Here's how the part is built. I have some questions about the finished solid (model axes, mm). Coordinates: 2 decimals unless noted, no trailing zeros. Write each loop counter-clockwise with the first axis right and the second up, starting at its lowest first coordinate (ties: lowest second). Pieces come first, ordered by that corner, then holes. Notation, with made-up numbers: M -24,56.25 L -13,56.25 A18 ccw -13,75.25 Z; hole C 31,32.5 d1. An arc over 180 degrees is marked long. Use one line per item in the form item = value. Start each with the question number.
1. I want a section at B-B, the plane y = 11. List the corners of the cut face in (x, z) for me.
2. I want a section at A-A, the plane x = 5. List the corners of the cut face in (y, z) for me, plus the area to 3 significant figures.
3. I want a section at C-C, the plane z = 2.5. List the corners of the cut face in (x, y) for me, plus the area to 3 significant figures.
4. I'm going to push a flat-ended pin straight in: pin 1 Ø3.5 at (y, z) = (5.5, 5) entering from +X. Where does the tip first touch, or does it pass through?
5. I want a section at D-D, the plane y = 7. List the corners of the cut face in (x, z) for me.
6. Please list where these lines run through material, in increasing order: line 1 along Y through (x, z) = (5, 2.5); line 2 along X through (y, z) = (8.25, 1.25); line 3 along X through (y, z) = (3, 2.75). Write a range as [from, to].
7. Thinking about a two-plate mould opening in Y: for faces 1 (the face through (21.97, 5.67, 2.81)), 2 (the face through (10, 16, 3)), 3 (the face through (24, 11, 4)), 4 (the face through (21.972, 10.425, 2.114)), which applies, released by +Y, released by -Y, zero draft, split by the parting line, or undercut?
from build123d import *

# Parameters (mm, degrees)
SKETCH1_W           = 20
SKETCH1_H           = 16
SKETCH1_R           = 1.65
BOSS_EXTRUDE1_DEPTH = 7
SKETCH2_R           = 1.5
BOSS_EXTRUDE2_DEPTH = 4


with BuildPart() as part:
    # Sketch1 → Boss-Extrude1 (new body)
    with BuildSketch(Plane.XY):
        with Locations((10, 8)):
            Rectangle(SKETCH1_W, SKETCH1_H)
        with Locations((5, 8)):
            Circle(SKETCH1_R, mode=Mode.SUBTRACT)
    extrude(amount=BOSS_EXTRUDE1_DEPTH)

    # Sketch2 → Boss-Extrude2 (add)
    with BuildSketch(Plane(origin=(20, 0, 0), x_dir=(0, 0, -1), z_dir=(1, 0, 0))):
        with Locations((-3.5, 7)):
            Circle(SKETCH2_R)
        with Locations((-3.5, 11)):
            Circle(SKETCH2_R)
    extrude(amount=BOSS_EXTRUDE2_DEPTH)


solid = part.part
Answer list:
q1.outline = M 0,0 L 20,0 L 20,2 L 24,2 L 24,5 L 20,5 L 20,7 L 0,7 Z
q2.outline = M 0,0 L 6.35,0 L 6.35,7 L 0,7 Z; M 9.65,0 L 16,0 L 16,7 L 9.65,7 Z
q2.area = 88.9 mm²
q3.outline = M 0,0 L 20,0 L 20,5.88 L 24,5.88 L 24,8.12 L 20,8.12 L 20,9.88 L 24,9.88 L 24,12.12 L 20,12.12 L 20,16 L 0,16 Z; hole C 5,8 d3.3
q3.area = 329 mm²
q4.pin_1 = 24
q5.outline = M 0,0 L 3.69,0 L 3.69,7 L 0,7 Z; M 6.31,0 L 20,0 L 20,2 L 24,2 L 24,5 L 20,5 L 20,7 L 6.31,7 Z
q6.line_1 = [0, 6.35], [9.65, 16]
q6.line_2 = [0, 3.37], [6.63, 20]
q6.line_3 = [0, 20]
q7.face_1 = undercut
q7.face_2 = released by +Y
q7.face_3 = zero draft
q7.face_4 = undercut
